from build123d import *

# Parameters (mm, degrees)
SKETCH2_R           = 10
SKETCH2_R_2         = 7.5
BOSS_EXTRUDE1_DEPTH = 8
BOSS_EXTRUDE2_START = -3
SKETCH3_R           = 13.75
SKETCH3_R_2         = 10
SKETCH3_R_3         = 7.5
BOSS_EXTRUDE2_DEPTH = 3
CHAMFER1_SIZE       = 1.5


with BuildPart() as part:
    # Sketch2 → Boss-Extrude1 (new body)
    with BuildSketch(Plane(origin=(0, 0, 0), x_dir=(1, 0, 0), z_dir=(0, 1, 0))):
        with Locations(Location((0, 0, 0), (0, 0, 270))):
            Circle(SKETCH2_R)
        with Locations(Location((0, 0, 0), (0, 0, 270))):
            Circle(SKETCH2_R_2, mode=Mode.SUBTRACT)
    extrude(amount=BOSS_EXTRUDE1_DEPTH)

    # Sketch3 → Boss-Extrude2 (add)
    # profile 1 of 2: a face of its own
    with BuildSketch(Plane(origin=(0, 0, 0), x_dir=(1, 0, 0), z_dir=(0, 1, 0)).offset(BOSS_EXTRUDE2_START)):
        with Locations(Location((0, 0, 0), (0, 0, 270))):
            Circle(SKETCH3_R)
        with Locations(Location((0, 0, 0), (0, 0, 270))):
            Circle(SKETCH3_R_2, mode=Mode.SUBTRACT)
    # profile 2 of 2: a face of its own
    with BuildSketch(Plane(origin=(0, 0, 0), x_dir=(1, 0, 0), z_dir=(0, 1, 0)).offset(BOSS_EXTRUDE2_START)):
        with Locations(Location((0, 0, 0), (0, 0, 270))):
            Circle(SKETCH3_R_2)
        with Locations(Location((0, 0, 0), (0, 0, 270))):
            Circle(SKETCH3_R_3, mode=Mode.SUBTRACT)
    extrude(amount=BOSS_EXTRUDE2_DEPTH)

    # Chamfer1
    chamfer1_edges = [part.edges().sort_by_distance(p)[0] for p in [
        (0, -3, -13.75),
        (0, -3, -7.5),
        (0, 8, -10),
    ]]
    chamfer(chamfer1_edges, length=CHAMFER1_SIZE)


solid = part.part
Source: CAD feature listing. Evaluate the final solid. Frame: model axes, mm. A direction names the side the tool comes from. Give positions to 0.01 mm unless a question says otherwise; leave off trailing zeros. Write each loop counter-clockwise with the first axis right and the second up, starting at its lowest first coordinate (ties: lowest second). Pieces come first, ordered by that corner, then holes. Notation, with made-up numbers: M 89,62 L 100,62 A7 ccw 100,72 Z; hole C -6,-29.75 d2. An arc over 180 degrees is marked long. Return JSON: item names as keys, results as strings. Group by question number.
1) Material intervals for line 1 along X through (y, z) = (3, 0); line 2 along X through (y, z) = (4, 5.75); line 3 along Z through (x, y) = (3, 6.25), sorted ascending. Write a range as [from, to].
2) Pull-direction query (X, two-part tool) for faces 1 (the face through (-12.2, -0.76, 6.34)), 2 (the face through (-10.12, 0, 0.95)), 3 (the face through (0.33, 3.183, -7.493)); classes: pulls with the +X half, pulls with the -X half, needs draft (parallel to the pull), parting line crosses it, or undercut.
3) Set-up query: faces 4 (the face through (-9.76, 3.2, -2.17)), 5 (the face through (6, -3, -7)). Return all of +Z, -Z, +X, -X, +Y, -Y with unobstructed straight access to the full face (end or side cutting, diameter ignored); none if empty.
4) Cut plane A-A, the plane x = 0. Output: boundary loops of the cut face in (y, z), plus the area to 4 significant figures.
5) Pin query (flat end, axial travel): P1, Ø3, axis at y = 3.5, z = 4, coming from the +X side; P2, Ø5, axis at x = -2.5, y = 6.5, coming from the +Z side; P3, Ø1.5, axis at y = 2.5, z = 1.5, coming from the -X side. Return the tip coordinate at first contact, or that it passes through.
6) Cut plane C-C, the plane y = 5. Output: boundary loops of the cut face in (x, z), plus the area to 3 significant figures.
7) Cut plane B-B, the plane z = 0. Output: boundary loops of the cut face in (x, y).
Recorded:
{
 "1": {"line 1": "x = [-10, -7.5], [7.5, 10]", "line 2": "x = [-8.18, -4.82], [4.82, 8.18]", "line 3": "z = [-9.54, -6.87], [6.87, 9.54]"},
 "2": {"face 1": "parting line crosses it", "face 2": "needs draft", "face 3": "undercut"},
 "3": {"face 4": "+Y", "face 5": "+Z, -Z, +X, -X, -Y"},
 "4": {"outline": "M -3,-12.25 L -1.5,-13.75 L 0,-13.75 L 0,-10 L 6.5,-10 L 8,-8.5 L 8,-7.5 L -1.5,-7.5 L -3,-9 Z; M -3,9 L -1.5,7.5 L 8,7.5 L 8,8.5 L 6.5,10 L 0,10 L 0,13.75 L -1.5,13.75 L -3,12.25 Z", "area": "70.75 mm²"},
 "5": {"P1": "stops at x = 9.68", "P2": "stops at z = 10", "P3": "stops at x = -9.97"},
 "6": {"outline": "C 0,0 d20; hole C 0,0 d15", "area": "137 mm²"},
 "7": {"outline": "M -13.75,-1.5 L -12.25,-3 L -9,-3 L -7.5,-1.5 L -7.5,8 L -8.5,8 L -10,6.5 L -10,0 L -13.75,0 Z; M 7.5,-1.5 L 9,-3 L 12.25,-3 L 13.75,-1.5 L 13.75,0 L 10,0 L 10,6.5 L 8.5,8 L 7.5,8 Z"}
}
